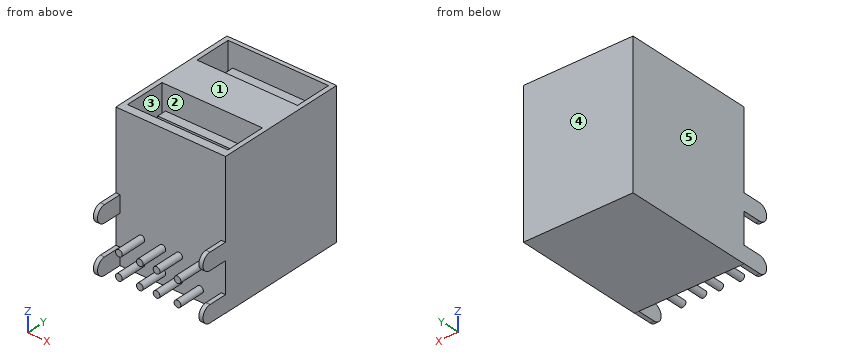
Autodesk Inventor part; units mm, degrees
ref_plane "YZ Plane" through (0, 0, 0) normal (1, 0, 0) x (0, 1, 0)
ref_plane "XZ Plane" through (0, 0, 0) normal (0, 1, 0) x (-1, 0, 0)
ref_plane "XY Plane" through (0, 0, 0) normal (0, 0, 1) x (1, 0, 0)
sketch "Sketch1" plane through (0, 0, 0) normal (0, 0, 1) x (1, 0, 0)
  line L0 (-6.55, 7.9) -> (6.55, 7.9)
  line L1 (6.55, 7.9) -> (6.55, -7.9)
  line L2 (6.55, -7.9) -> (-6.55, -7.9)
  line L3 (-6.55, -7.9) -> (-6.55, 7.9)
  point P0 (0, 0)
  dimension "d0" = 13.1
  dimension "d1" = 15.8
  dimension "d2" = 7.9
  dimension "d3" = 6.55
extrude "Extrusion1" add sketch "Sketch1" along normal blind 17
sketch "Sketch2" plane through (0, 0, 17) normal (0, 0, 1) x (1, 0, 0)
  line L0 (-6, 7.4) -> (6, 7.4)
  line L1 (6, 7.4) -> (6, 3)
  line L2 (6, 3) -> (-6, 3)
  line L3 (-6, 3) -> (-6, 7.4)
  line L4 (-6, -2) -> (6, -2)
  line L5 (6, -2) -> (6, -6.9)
  line L6 (6, -6.9) -> (-6, -6.9)
  line L7 (-6, -6.9) -> (-6, -2)
  line L8 (-6.55, -7.9) -> (6.55, -7.9)
  line L9 (6.55, 7.9) -> (-6.55, 7.9)
  point P0 (0, 0)
  dimension "d6" = 12
  dimension "d7" = 12
  dimension "d8" = 6
  dimension "d9" = 1
  dimension "d10" = 0.5
  dimension "d11" = 5
  dimension "d12" = 2
extrude "Extrusion2" cut sketch "Sketch2" against normal blind 10
sketch "Sketch3" plane through (0, 0, 7) normal (0, 0, 1) x (1, 0, 0)
  line L0 (-4.6506, 6.4578) -> (5.055, 6.4578)
  line L1 (5.055, 6.4578) -> (5.055, 5.3457)
  line L2 (5.055, 5.3457) -> (-4.6506, 5.3457)
  line L3 (-4.6506, 5.3457) -> (-4.6506, 6.4578)
  line L4 (-4.6506, -3.0962) -> (5.055, -3.0962)
  line L5 (5.055, -3.0962) -> (5.055, -4.2083)
  line L6 (5.055, -4.2083) -> (-4.6506, -4.2083)
  line L7 (-4.6506, -4.2083) -> (-4.6506, -3.0962)
  point P0 (0, 0)
extrude "Extrusion3" add sketch "Sketch3" along normal blind 8
sketch "Sketch4" plane through (6.55, -7.9, 0) normal (1, 0, 0) x (0, 0, -1)
  line L0 (-7.7, 2.838) -> (-5.7, 2.838)
  line L1 (-5.7, 2.838) -> (-5.7, -3.2)
  line L2 (-5.7, -3.2) -> (-7.7, -3.2)
  line L3 (-7.7, -3.2) -> (-7.7, 2.838)
  line L4 (-17, 0) -> (-17, 15.8)
  line L5 (-2.02, 6.1684) -> (-0.02, 6.1684)
  line L6 (-0.02, 6.1684) -> (-0.02, -3.2)
  line L7 (-0.02, -3.2) -> (-2.02, -3.2)
  line L8 (-2.02, -3.2) -> (-2.02, 6.1684)
  arc A0 (-7.7, -2.2) -> (-5.7, -2.2) centre (-6.7, -2.2) ccw
  arc A1 (-2.02, -2.2) -> (-0.02, -2.2) centre (-1.02, -2.2) ccw
  point P0 (0, 7.9)
  dimension "d17" = 2
  dimension "d18" = 9.3
  dimension "d19" = 2
  dimension "d20" = 3.68
  dimension "d21" = 3.2
  dimension "d22" = 0
extrude "Extrusion4" add sketch "Sketch4" against normal blind 0.5 contours L0 L1 A0 L3 | L5 L6 A1 L8
sketch "Sketch5" plane through (-6.55, -7.9, 0) normal (0, -1, 0) x (1, 0, 0)
  line L0 (13.8244, 1.33) -> (1.8735, 1.33) construction
  line L1 (13.8244, 3.95) -> (1.8735, 3.95) construction
  line L2 (13.1, 7.7) -> (12.6, 7.7)
  circle A0 centre (5.55, 1.33) radius 0.4
  circle A1 centre (5.55, 3.95) radius 0.4
  circle A2 centre (7.55, 1.33) radius 0.4
  circle A3 centre (7.55, 3.95) radius 0.4
  circle A4 centre (3.05, 1.33) radius 0.4
  circle A5 centre (3.05, 3.95) radius 0.4
  circle A6 centre (10.05, 3.95) radius 0.4
  circle A7 centre (10.05, 1.33) radius 0.4
  point P0 (6.55, 0)
  dimension "d25" = 2.62
  dimension "d26" = 3.75
  dimension "d27" = 2
  dimension "d28" = 1
  dimension "d29" = 2
  dimension "d30" = 1
  dimension "d31" = 2.5
  dimension "d32" = 2.5
  dimension "d33" = 2.5
  dimension "d34" = 2.5
  dimension "d35" = 0.8
  dimension "d36" = 0.8
  dimension "d37" = 0.8
  dimension "d38" = 0.8
  dimension "d39" = 0.8
  dimension "d40" = 0.8
  dimension "d41" = 0.8
  dimension "d42" = 0.8
extrude "Extrusion5" add sketch "Sketch5" along normal blind 3.2
mirror "Mirror1" about plane through (0, 0, 0) normal (1, 0, 0) of "Extrusion4"
properties part number "USBA_Stack"
Source: CAD feature listing. Evaluate the final solid. Frame: model axes, mm. Face numbers are marked on the shaded views. A direction names the side the tool comes from. Give positions to 0.01 mm unless a question says otherwise; leave off trailing zeros. Loops run counter-clockwise (first coordinate to the right, second up) from the corner with the lowest first, then second, coordinate; pieces in that order, holes last. Notation, with made-up numbers: (-19, -29) -> (-9, -29) arc R24 cw to (-9, -12) -> close; hole circle Ø8 at (5, 10). An arc over 180 degrees is marked (long way). Put each result on its own line as item: value. Start each with the question number.
1) Contact query for flat-ended pins moving along their axis: P1, Ø0.6, axis at x = -6, y = -9, coming from the +Z side; P2, Ø3, axis at x = 0, z = 7.5, coming from the -Y side; P3, Ø0.9, axis at x = -1.5, y = -3.5, coming from the +Z side. Output: stop coordinate, or through.
2) Draft query along Y for the marked faces 3, 4 and 5. Return one class per face: released by +Y, released by -Y, zero draft, split by the parting line, or undercut.
3) Reachability of the marked faces 1 and 2 from +Z, -Z, +X, -X, +Y, -Y: full face, straight path, thin tool, end or side. Return the list, or none.
4) Cut plane D-D (y = -3.5). Return loops of the section in (x, z) (3 decimals).
5) Cut plane C-C (z = 3.95). Return loops of the section in (x, y).
6) Cut plane A-A (z = 8.75). Return loops of the section in (x, y) (3 decimals).
7) Material intervals for probe 1 along X at (y, z) = (-3.75, 7.5) (3 decimals); probe 2 along Y at (x, z) = (0.5, 14.5); probe 3 along Y at (x, z) = (-5.5, 12.5), sorted ascending.
8) Cut plane B-B (x = 0.25). Return loops of the section in (y, z), then the cut area to 3 significant figures.
Results are:
1. P1: stops at z = 7.7
1. P2: stops at y = -7.9
1. P3: stops at z = 15
2. face 3: undercut
2. face 4: released by +Y
2. face 5: zero draft
3. face 1: +Z, +X, -X, +Y, -Y
3. face 2: +Z
4. outline: (-6.55, 0) -> (6.55, 0) -> (6.55, 17) -> (6, 17) -> (6, 7) -> (5.055, 7) -> (5.055, 15) -> (-4.651, 15) -> (-4.651, 7) -> (-6, 7) -> (-6, 17) -> (-6.55, 17) -> close
5. outline: (-6.55, -7.9) -> (-3.9, -7.9) -> (-3.9, -11.1) -> (-3.1, -11.1) -> (-3.1, -7.9) -> (-1.4, -7.9) -> (-1.4, -11.1) -> (-0.6, -11.1) -> (-0.6, -7.9) -> (0.6, -7.9) -> (0.6, -11.1) -> (1.4, -11.1) -> (1.4, -7.9) -> (3.1, -7.9) -> (3.1, -11.1) -> (3.9, -11.1) -> (3.9, -7.9) -> (6.55, -7.9) -> (6.55, 7.9) -> (-6.55, 7.9) -> close
6. outline: (-6.55, -7.9) -> (6.55, -7.9) -> (6.55, 7.9) -> (-6.55, 7.9) -> close; (-4.651, -4.208) -> (5.055, -4.208) -> (5.055, -3.096) -> (-4.651, -3.096) -> close; (-4.651, 5.346) -> (5.055, 5.346) -> (5.055, 6.458) -> (-4.651, 6.458) -> close; hole (-6, -6.9) -> (6, -6.9) -> (6, -2) -> (-6, -2) -> close; hole (-6, 3) -> (6, 3) -> (6, 7.4) -> (-6, 7.4) -> close
7. probe 1: x = -6.55 to -6, -4.651 to 5.055, 6 to 6.55
7. probe 2: y = -7.9 to -6.9, -4.21 to -3.1, -2 to 3, 5.35 to 6.46, 7.4 to 7.9
7. probe 3: y = -7.9 to -6.9, -2 to 3, 7.4 to 7.9
8. outline: (-7.9, 0) -> (7.9, 0) -> (7.9, 17) -> (7.4, 17) -> (7.4, 7) -> (6.46, 7) -> (6.46, 15) -> (5.35, 15) -> (5.35, 7) -> (3, 7) -> (3, 17) -> (-2, 17) -> (-2, 7) -> (-3.1, 7) -> (-3.1, 15) -> (-4.21, 15) -> (-4.21, 7) -> (-6.9, 7) -> (-6.9, 17) -> (-7.9, 17) -> close
8. area: 193 mm2
